Source: CAD feature listing. Evaluate the final solid. Frame: model axes, mm. A direction names the side the tool comes from. Give positions to 0.01 mm unless a question says otherwise; leave off trailing zeros. Write each loop counter-clockwise with the first axis right and the second up, starting at its lowest first coordinate (ties: lowest second). Pieces come first, ordered by that corner, then holes. Notation, with made-up numbers: M 33.25,-28.75 L 73.25,-28.75 A13 cw 73.25,-23.75 Z; hole C 35,-13 d8. An arc over 180 degrees is marked long. Return JSON: item names as keys, results as strings.
```python
from build123d import *

# Parameters (mm, degrees)
SKETCH2_R           = 1.95
BOSS_EXTRUDE1_DEPTH = 34
SKETCH3_R           = 3.75
BOSS_EXTRUDE2_DEPTH = 2.5
SKETCH4_W           = 2
SKETCH4_H           = 10
CUT_EXTRUDE1_DEPTH  = 1.5
FILLET1_R           = 0.2
CHAMFER1_SIZE       = 0.5


with BuildPart() as part:
    # Sketch2 → Boss-Extrude1 (new body)
    with BuildSketch(Plane.XY):
        Circle(SKETCH2_R)
    extrude(amount=BOSS_EXTRUDE1_DEPTH)

    # Sketch3 → Boss-Extrude2 (add)
    with BuildSketch(Plane(origin=(0, 0, 0), x_dir=(-1, 0, 0), z_dir=(0, 0, -1))):
        Circle(SKETCH3_R)
    extrude(amount=BOSS_EXTRUDE2_DEPTH)

    # Sketch4 → Cut-Extrude1 (cut)
    with BuildSketch(Plane(origin=(0, 0, -2.5), x_dir=(-1, 0, 0), z_dir=(0, 0, -1))):
        Rectangle(SKETCH4_W, SKETCH4_H)
    extrude(amount=-CUT_EXTRUDE1_DEPTH, mode=Mode.SUBTRACT)

    # Fillet1
    fillet1_edges = [part.edges().sort_by_distance(p)[0] for p in [
        (-2.984334097, 2.270737766, -2.5),
        (3.75, 0, 0),
        (3.75, 0, -2.5),
    ]]
    fillet(fillet1_edges, radius=FILLET1_R)

    # Chamfer1
    chamfer1_edges = [part.edges().sort_by_distance(p)[0] for p in [
        (-1.95, 0, 34),
    ]]
    chamfer(chamfer1_edges, length=CHAMFER1_SIZE)


solid = part.part
```
1) Set-up query: faces 1 (the face through (-2, 0, -2.5)), 2 (the face through (-1.437, 1.318, 16.516)), 3 (the face through (1, 0, -2)). Return all of +Z, -Z, +X, -X, +Y, -Y with unobstructed straight access to the full face (end or side cutting, diameter ignored); none if empty.
Numbers:
{"face 1": "-Z, +X, -X, +Y, -Y", "face 2": "+Z", "face 3": "-Z, +Y, -Y"}
2) Contact query for flat-ended pins moving along their axis: pin 1 Ø1 at (y, z) = (-0.5, 4.5) entering from -X; pin 2 Ø3 at (y, z) = (2.5, 16) entering from -X; pin 3 Ø1.6 at (x, y) = (0, -1) entering from -Z. Output: stop coordinate, or through.
Numbers:
{"pin 1": "stops at x = -1.95", "pin 2": "stops at x = -1.67", "pin 3": "stops at z = -1"}
3) Line query: line 1 (Z direction, x = 1.75, y = -1); line 2 (Z direction, x = -0.25, y = 0.5); line 3 (Y direction, x = -0.5, z = 17.5). Output: solid intervals per line, ascending. Write a range as [from, to].
Numbers:
{"line 1": "z = [-2.5, 0]", "line 2": "z = [-1, 34]", "line 3": "y = [-1.88, 1.88]"}
4) Cut plane A-A, the plane x = 0. Return the cut outline in (y, z).
Numbers:
{"outline": "M -3.75,-1 L 3.75,-1 L 3.75,-0.2 A0.2 ccw 3.55,0 L 1.95,0 L 1.95,33.5 L 1.45,34 L -1.45,34 L -1.95,33.5 L -1.95,0 L -3.55,0 A0.2 ccw -3.75,-0.2 Z"}
5) Cut plane C-C, the plane z = 7. Return the cut outline in (x, y), then the cut area to 3 significant figures.
Numbers:
{"outline": "C 0,0 d3.9", "area": "11.9 mm²"}
6) Cut plane B-B, the plane y = 0. Return the cut outline in (x, z).
Numbers:
{"outline": "M -3.75,-2.3 A0.2 ccw -3.55,-2.5 L -1,-2.5 L -1,-1 L 1,-1 L 1,-2.5 L 3.55,-2.5 A0.2 ccw 3.75,-2.3 L 3.75,-0.2 A0.2 ccw 3.55,0 L 1.95,0 L 1.95,33.5 L 1.45,34 L -1.45,34 L -1.95,33.5 L -1.95,0 L -3.55,0 A0.2 ccw -3.75,-0.2 Z"}
7) Draft query along X for faces 4 (the face through (0, 0, -1)), 5 (the face through (-1, 0, -2)), 6 (the face through (-3.577, 1.126, -1.235)), 7 (the face through (-2, -2, 0)). Return one class per face: released by +X, released by -X, zero draft, split by the parting line, or undercut.
Numbers:
{"face 4": "undercut", "face 5": "undercut", "face 6": "split by the parting line", "face 7": "zero draft"}
